Could you check a few things on this model? Use its own coordinates, in mm. Face numbers are marked on the shaded views. A direction names the side the tool comes from. Coordinates: 2 decimals unless noted, no trailing zeros. Loops run counter-clockwise (first coordinate to the right, second up) from the corner with the lowest first, then second, coordinate; pieces in that order, holes last.
1) Imagine slicing it at C-C on x = -671. Please give me the cut outline in (y, z).
2) Imagine slicing it at D-D on y = 183.5. Please give me the cut outline in (x, z), plus the area to 3 significant figures.
3) Imagine slicing it at B-B on z = 7.75. Give the number of separate pieces and of enclosed holes in the cut face, plus the area to 3 significant figures.
4) If I drill on line 1 along Y through (x, z) = (-621, 8); line 2 along Y through (x, z) = (-639, 4); line 3 along Y through (x, z) = (-622, 6.75), over which ranges is the centre line in solid material (lowest first)?
5) Thinking about a two-plate mould opening in X: for the marked faces 6, 7, 8 and 9, which applies, released by +X, released by -X, zero draft, split by the parting line, or undercut?
6) Imagine slicing it at A-A on y = 114. Please give me the cut outline in (x, z), plus the area to 3 significant figures.
7) For the marked faces 1, 2, 3, 4 and 5, which set-ups out of +Z, -Z, +X, -X, +Y, -Y let a thin tool reach every point of the face, with its end or its side?
8) Will these pins go through, and if not, where does the flat tip stop? P1, Ø6, axis at y = 142, z = 1.5, coming from the -X side; P2, Ø1.9, axis at x = -612, y = 148, coming from the +Z side; P3, Ø9.5, axis at x = -620.67, y = 147.96, coming from the +Z side; P4, Ø5, axis at x = -612.66, y = 147.96, coming from the +Z side (3 decimals).
```python
from build123d import *

# Parameters (mm, degrees)
F0_R     = 63.5
F0_R_2   = 25.4
F0_R_3   = 2.032
F0_R_4   = 4.064
F1_DEPTH = 12.7
F2_R     = 3.175
F2_R_2   = 2.032
F3_DEPTH = 9.525
F4_DEPTH = 12.7


with BuildPart() as f1:
    # F0 (on Top) → F1 (new body)
    with BuildSketch(Plane.XY):
        with Locations((-620.6655502319, 147.9596942663)):
            Circle(F0_R)
        with Locations((-620.6655502319, 147.9596942663)):
            Circle(F0_R_2, mode=Mode.SUBTRACT)
        with Locations((-620.6655502319, 147.9596942663)):
            Circle(F0_R_2)
        with Locations((-620.6655502319, 139.9586942663)):
            Circle(F0_R_3, mode=Mode.SUBTRACT)
        with Locations((-628.6665502319, 147.9596942663)):
            Circle(F0_R_3, mode=Mode.SUBTRACT)
        with Locations((-620.6655502319, 147.9596942663)):
            Circle(F0_R_4, mode=Mode.SUBTRACT)
        with Locations((-612.6645502319, 147.9596942663)):
            Circle(F0_R_3, mode=Mode.SUBTRACT)
        with Locations((-620.6655502319, 155.9606942663)):
            Circle(F0_R_3, mode=Mode.SUBTRACT)
    extrude(amount=F1_DEPTH)

    # F2 (on face) → F3 (cut)
    with BuildSketch(Plane.XY.offset(12.7)):
        with Locations((-628.6665502319, 147.9596942663)):
            Circle(F2_R)
        with Locations((-628.6665502319, 147.9596942663)):
            Circle(F2_R_2, mode=Mode.SUBTRACT)
        with BuildLine():
            ThreePointArc((-620.6655502319, 159.1356942663), (-622.9106142622, 153.7156302361), (-617.4905502319, 155.9606942663))
            ThreePointArc((-617.4905502319, 155.9606942663), (-618.4204862017, 158.2057582966), (-620.6655502319, 159.1356942663))
        make_face()
        with BuildLine():
            ThreePointArc((-618.6335502319, 155.9606942663), (-622.1023912113, 154.5238532869), (-620.6655502319, 157.9926942663))
            ThreePointArc((-620.6655502319, 157.9926942663), (-619.2287092526, 157.3975352457), (-618.6335502319, 155.9606942663))
        make_face(mode=Mode.SUBTRACT)
        with Locations((-612.6645502319, 147.9596942663)):
            Circle(F2_R)
        with Locations((-612.6645502319, 147.9596942663)):
            Circle(F2_R_2, mode=Mode.SUBTRACT)
        with Locations((-620.6655502319, 139.9586942663)):
            Circle(F2_R)
        with Locations((-620.6655502319, 139.9586942663)):
            Circle(F2_R_2, mode=Mode.SUBTRACT)
    extrude(amount=-F3_DEPTH, mode=Mode.SUBTRACT)

    # F2 (on face) → F4 (cut)
    with BuildSketch(Plane.XY.offset(12.7)):
        with BuildLine():
            ThreePointArc((-628.7935502319, 173.3596942663), (-625.8046499913, 168.8251534834), (-620.6655502319, 167.0686688056))
            ThreePointArc((-620.6655502319, 167.0686688056), (-615.5264504725, 168.8251534834), (-612.5375502319, 173.3596942663))
            ThreePointArc((-612.5375502319, 173.3596942663), (-608.9080068362, 191.8026056382), (-598.5370363488, 207.4792614129))
            ThreePointArc((-598.5370363488, 207.4792614129), (-620.6796633161, 211.459692698), (-642.8205187681, 207.4694192628))
            ThreePointArc((-642.8205187681, 207.4694192628), (-632.4371990863, 191.8003367826), (-628.7935502319, 173.3596942663))
        make_face()
        with BuildLine():
            ThreePointArc((-638.5985954881, 167.6987487483), (-652.755853558, 180.063481219), (-661.1467504616, 196.8833330105))
            ThreePointArc((-661.1467504616, 196.8833330105), (-675.6652185561, 179.6974711927), (-683.2799681192, 158.5277911922))
            ThreePointArc((-683.2799681192, 158.5277911922), (-664.5184847964, 159.6854685722), (-646.7265954881, 153.6206397844))
            ThreePointArc((-646.7265954881, 153.6206397844), (-637.2144076232, 157.5141815359), (-638.5985954881, 167.6987487483))
        make_face()
        with BuildLine():
            ThreePointArc((-646.7265954881, 142.2987487483), (-664.5133969537, 136.2205698472), (-683.2752643448, 137.3637658638))
            ThreePointArc((-683.2752643448, 137.3637658638), (-675.6511054719, 116.197472761), (-661.1249995831, 99.0180661957))
            ThreePointArc((-661.1249995831, 99.0180661957), (-652.7468359421, 115.8448260559), (-638.5985954881, 128.2206397844))
            ThreePointArc((-638.5985954881, 128.2206397844), (-637.2144076232, 138.4052069967), (-646.7265954881, 142.2987487483))
        make_face()
        with BuildLine():
            ThreePointArc((-628.7935502319, 122.5596942663), (-632.4230936276, 104.1167828944), (-642.7940641151, 88.4401271197))
            ThreePointArc((-642.7940641151, 88.4401271197), (-620.6514371477, 84.4596958347), (-598.5105816958, 88.4499692698))
            ThreePointArc((-598.5105816958, 88.4499692698), (-608.8939013776, 104.11905175), (-612.5375502319, 122.5596942663))
            ThreePointArc((-612.5375502319, 122.5596942663), (-620.6655502319, 128.8507197271), (-628.7935502319, 122.5596942663))
        make_face()
        with BuildLine():
            ThreePointArc((-580.1843500023, 99.0360555222), (-565.6658819077, 116.2219173399), (-558.0511323446, 137.3915973404))
            ThreePointArc((-558.0511323446, 137.3915973404), (-576.8126156674, 136.2339199605), (-594.6045049758, 142.2987487483))
            ThreePointArc((-594.6045049758, 142.2987487483), (-604.1166928407, 138.4052069967), (-602.7325049758, 128.2206397844))
            ThreePointArc((-602.7325049758, 128.2206397844), (-588.5752469059, 115.8559073136), (-580.1843500023, 99.0360555222))
        make_face()
        with BuildLine():
            ThreePointArc((-558.0558361191, 158.5556226688), (-565.6799949919, 179.7219157716), (-580.2061008808, 196.9013223369))
            ThreePointArc((-580.2061008808, 196.9013223369), (-588.5842645218, 180.0745624768), (-602.7325049758, 167.6987487483))
            ThreePointArc((-602.7325049758, 167.6987487483), (-604.1166928407, 157.5141815359), (-594.6045049758, 153.6206397844))
            ThreePointArc((-594.6045049758, 153.6206397844), (-576.8177035102, 159.6988186855), (-558.0558361191, 158.5556226688))
        make_face()
    extrude(amount=-F4_DEPTH, mode=Mode.SUBTRACT)


solid = f1.part
```
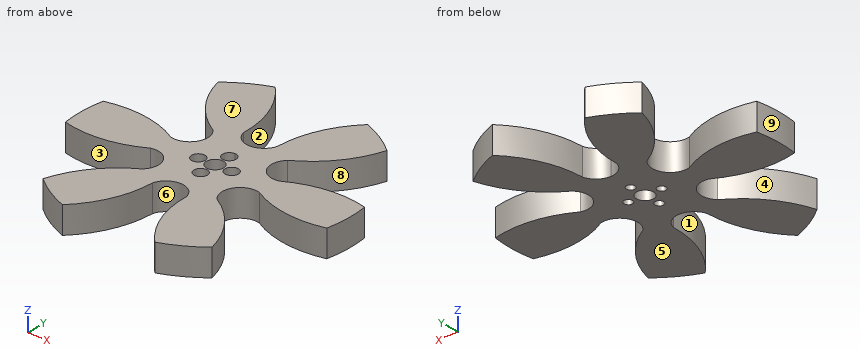
Filled in:
1. outline: (135.78, 0) - (160.12, 0) - (160.12, 12.7) - (135.78, 12.7) - close
2. outline: (-655.18, 0) - (-629.87, 0) - (-629.87, 12.7) - (-655.18, 12.7) - close; (-611.47, 0) - (-586.17, 0) - (-586.17, 12.7) - (-611.47, 12.7) - close
2. area: 643 mm2
3. separate pieces: 1
3. enclosed holes: 5
3. area: 6,210 mm2
4. line 1: y = 128.84 to 136.8, 143.12 to 143.91, 152.01 to 152.8, 159.12 to 167.08
4. line 2: y = 92.76 to 127.99, 140.56 to 155.36, 167.93 to 203.12
4. line 3: y = 128.74 to 137.08, 142.84 to 144.12, 151.8 to 153.08, 158.84 to 167.18
5. face 6: undercut
5. face 7: zero draft
5. face 8: released by +X
5. face 9: released by -X
6. outline: (-654.1, 0) - (-629.55, 0) - (-629.55, 12.7) - (-654.1, 12.7) - close; (-611.78, 0) - (-587.21, 0) - (-587.21, 12.7) - (-611.78, 12.7) - close
6. area: 624 mm2
7. face 1: +Z, -Z, -Y
7. face 2: +Z, -Z, +Y
7. face 3: +Z, -Z
7. face 4: +Z, -Z, -X
7. face 5: -Z, +X, -X, +Y, -Y
8. P1: stops at x = -684.1
8. P2: passes through
8. P3: stops at z = 12.7
8. P4: stops at z = 3.175
